Input: part model. Units: mm. Frame: model coordinates. Face numbers are marked on the shaded views. A direction names the side the tool comes from. Coordinates: 2 decimals unless noted, no trailing zeros. Loops run counter-clockwise (first coordinate to the right, second up) from the corner with the lowest first, then second, coordinate; pieces in that order, holes last. Notation, with made-up numbers: (77.5, 83) - (135.5, 83) arc R22 ccw to (135.5, 121) - close; hole circle Ø9 at (55.5, 17.5). An arc over 180 degrees is marked (long way). Use a Markdown table: item, result. Add a question column.
1. Draft query along Z for the marked faces 5, 6 and 7. Return one class per face: released by +Z, released by -Z, zero draft, split by the parting line, or undercut.
2. Contact query for flat-ended pins moving along their axis: P1, Ø8, axis at y = 1.5, z = 11.5, coming from the +X side; P2, Ø4, axis at y = -5.5, z = 166.5, coming from the +X side; P3, Ø10, axis at y = -6.5, z = 44.5, coming from the +X side. Output: stop coordinate, or through.
3. Section query A-A on y = -7. Return the cut outline in (x, z).
4. Section query C-C on z = 46. Return the cut outline in (x, y), then the cut area to 3 significant figures.
5. Ray query, L1, parallel to Z at x = 36.5, y = -3; L2, parallel to Y at x = 4, z = 93.5; L3, parallel to X at y = -5, z = 123. Return the intervals inside material, ascending. Write a range as [from, to].
6. Section query B-B on x = 11.5. Return the cut outline in (y, z) (3 decimals), then the cut area to 3 significant figures.
7. Section query D-D on x = 51. Return the cut outline in (y, z) (3 decimals).
8. Access query for the marked faces 1, 2, 3 and 4. Directions: +Z, -Z, +X, -X, +Y, -Y. A direction counts if a zero-diameter tool reaches every point of the face in a straight line with its end or side. Return the directions, or none.
```python
from build123d import *

# Parameters (mm, degrees)
F1_DEPTH  = 12.7
F3_DEPTH  = 38.1
F4_W      = 14.7766079754
F4_H      = 8.8374735788
F5_DEPTH  = 3.175
F7_DEPTH  = 66.675
F8_W      = 12.7
F8_H      = 19.4
F9_DEPTH  = 66.548
F10_DEPTH = 34.925
F11_W     = 34.925
F11_H     = 31.75
F12_DEPTH = 25.4
F13_W     = 3.175
F13_H     = 31.75
F14_DEPTH = 25.4
F15_DEPTH = 3.175
F17_DEPTH = 8.128
F19_DEPTH = 0.381


with BuildPart() as f1:
    # F0 (on Front) → F1 (new body)
    with BuildSketch(Plane.XZ):
        Polygon((0, 173.39), (0, 0), (38.1, 0), (38.1, 19.4), (25.4, 19.4), (25.4, 79.73), (38.1, 79.73), (38.1, 130.53), (25.4, 130.53), (25.4, 147.99), (38.1, 147.99), (38.1, 173.39), align=None)
    extrude(amount=F1_DEPTH)

    # F2 (on face) → F3 (join)
    with BuildSketch(Plane.YZ.offset(38.1)):
        Polygon((0, -7.62), (-2.7734531851, 0), (-9.9265468149, 0), (-12.7, -7.62), align=None)
    extrude(amount=-F3_DEPTH)

    # F4 (on face) → F5 (cut)
    with BuildSketch(Plane(origin=(0, 0, 0), x_dir=(0, -1, 0), z_dir=(-1, 0, 0))):
        with Locations((7.3883039877, -4.4187367894)):
            Rectangle(F4_W, F4_H)
    extrude(amount=-F5_DEPTH, mode=Mode.SUBTRACT)

    # F6 (on face) → F7 (join)
    with BuildSketch(Plane.YZ.offset(38.1)):
        Polygon((-12.7, -7.62), (-9.9265468149, 0), (-12.7, 0), (-19.4515468149, 0), (-22.225, -7.62), align=None)
        Polygon((0, -7.62), (-2.7734531851, 0), (-9.9265468149, 0), (-12.7, -7.62), align=None)
        Polygon((-2.7734531851, 0), (0, 0), (0, 19.4), (-12.7, 19.4), (-12.7, 0), (-9.9265468149, 0), align=None)
        Polygon((6.7515468149, 0), (0, 0), (-2.7734531851, 0), (0, -7.62), (9.525, -7.62), align=None)
    extrude(amount=F7_DEPTH)

    # F8 (on face) → F9 (cut)
    with BuildSketch(Plane.YZ.offset(104.775)):
        with Locations((-6.35, 9.7)):
            Rectangle(F8_W, F8_H)
    extrude(amount=-F9_DEPTH, mode=Mode.SUBTRACT)

    # F6 (on face) → F10 (join)
    with BuildSketch(Plane.YZ.offset(38.1)):
        Polygon((6.7515468149, 0), (0, 0), (-2.7734531851, 0), (0, -7.62), (9.525, -7.62), align=None)
        Polygon((-12.7, -7.62), (-9.9265468149, 0), (-12.7, 0), (-19.4515468149, 0), (-22.225, -7.62), align=None)
    extrude(amount=-F10_DEPTH)

    # F11 (on face) → F12 (cut)
    with BuildSketch(Plane(origin=(0, 0, -7.62), x_dir=(1, 0, 0), z_dir=(0, 0, -1))):
        with Locations((87.3125, 6.35)):
            Rectangle(F11_W, F11_H)
    extrude(amount=-F12_DEPTH, mode=Mode.SUBTRACT)

    # F13 (on face) → F14 (cut)
    with BuildSketch(Plane(origin=(0, 0, -7.62), x_dir=(1, 0, 0), z_dir=(0, 0, -1))):
        with Locations((68.2625, 6.35)):
            Rectangle(F13_W, F13_H)
    extrude(amount=-F14_DEPTH, mode=Mode.SUBTRACT)

    # F15 (add): a face of the model
    f15_faces = [f1.faces().sort_by_distance(p)[0] for p in [
        (3.175, -6.35, -3.9315564286),
    ]]
    extrude(f15_faces, amount=F15_DEPTH)

    # F16 (on face) → F17 (cut)
    with BuildSketch(Plane.XY):
        Polygon((43.9181570547, 6.7515468149), (40.194484, -9.3774531851), (60.325, -9.3774531851), (56.6013269453, 6.7515468149), align=None)
        Polygon((40.194484, 22.8805468149), (43.9181570547, 6.7515468149), (56.6013269453, 6.7515468149), (60.325, 22.8805468149), align=None)
    extrude(amount=-F17_DEPTH, mode=Mode.SUBTRACT)

    # F18 (on face) → F19 (cut)
    with BuildSketch(Plane.YZ.offset(66.675)):
        Polygon((-19.4515468149, 0), (-22.225, -7.62), (9.525, -7.62), (6.7515468149, 0), align=None)
    extrude(amount=-F19_DEPTH, mode=Mode.SUBTRACT)


solid = f1.part
```
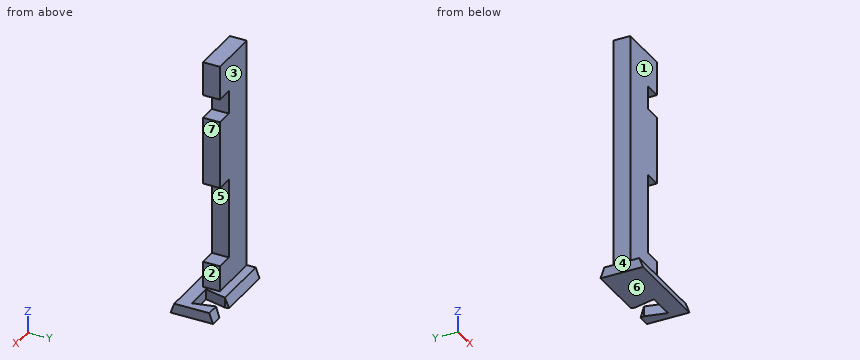
Resolved:
| question | item | result |
|---|---|---|
| 1 | face 5 | undercut |
| 1 | face 6 | released by -Z |
| 1 | face 7 | zero draft |
| 2 | P1 | x = 38.23 |
| 2 | P2 | x = 38.1 |
| 2 | P3 | x = 25.4 |
| 3 | outline | (0, -7.62) - (40.74, -7.62) - (40.74, 0) - (38.23, 0) - (38.23, 19.4) - (25.4, 19.4) - (25.4, 79.73) - (38.1, 79.73) - (38.1, 130.53) - (25.4, 130.53) - (25.4, 147.99) - (38.1, 147.99) - (38.1, 173.39) - (0, 173.39) - close; (59.78, -7.62) - (66.29, -7.62) - (66.29, 0) - (59.78, 0) - close |
| 4 | outline | (0, -12.7) - (25.4, -12.7) - (25.4, 0) - (0, 0) - close |
| 4 | area | 323 mm² |
| 5 | L1 | [-7.62, 19.4], [79.73, 130.53], [147.99, 173.39] |
| 5 | L2 | [-12.7, 0] |
| 5 | L3 | [0, 38.1] |
| 6 | outline | (-22.225, -7.62) - (9.525, -7.62) - (6.752, 0) - (0, 0) - (0, 173.39) - (-12.7, 173.39) - (-12.7, 0) - (-19.452, 0) - close |
| 6 | area | 2,420 mm² |
| 7 | outline | (-22.225, -7.62) - (-9.377, -7.62) - (-9.377, 0) - (-19.452, 0) - close |
| 8 | face 1 | +Z, +X, -X, -Y |
| 8 | face 2 | +Z, +X, +Y, -Y |
| 8 | face 3 | +Z, +X, -X, +Y |
| 8 | face 4 | +Z, -Z, -X, +Y, -Y |
